Autodesk Inventor part; units mm, degrees
ref_plane "YZ Plane" through (0, 0, 0) normal (1, 0, 0) x (0, 1, 0)
ref_plane "XZ Plane" through (0, 0, 0) normal (0, 1, 0) x (-1, 0, 0)
ref_plane "XY Plane" through (0, 0, 0) normal (0, 0, 1) x (1, 0, 0)
sketch "スケッチ1" plane through (0, 0, 0) normal (0, 0, 1) x (1, 0, 0)
  line L0 (-17.75, 4) -> (17.75, 4)
  line L1 (17.75, 4) -> (17.75, -4)
  line L2 (17.75, -4) -> (-17.75, -4)
  line L3 (-17.75, -4) -> (-17.75, 4)
  line L4 (-17.75, 4) -> (17.75, -4) construction
  line L5 (17.75, 4) -> (-17.75, -4) construction
  point P0 (0, 0)
  dimension "d0" = 35.5
  dimension "d1" = 8
extrude "押し出し1" add sketch "スケッチ1" along normal mid plane 0.55
sketch "スケッチ2" plane through (0, 0, 0.275) normal (0, 0, 1) x (1, 0, 0)
  line L0 (9.6635, 0) -> (12.3865, 0) construction
  line L1 (9.6635, 1.3635) -> (12.3865, 1.3635)
  line L2 (12.3865, -1.3635) -> (9.6635, -1.3635)
  arc A0 (9.6635, 1.3635) -> (9.6635, -1.3635) centre (9.6635, 0) ccw
  arc A1 (12.3865, -1.3635) -> (12.3865, 1.3635) centre (12.3865, 0) ccw
  line L3 (17.75, -4) -> (17.75, 4)
  line L4 (17.75, 4) -> (-17.75, 4)
  point P0 (0, 0)
  point P1 (11.025, 0)
  point P2 (13.75, 0)
  point P3 (8.3, 0)
  dimension "d4" = 2.727
  dimension "d5" = 5.45
  dimension "d6" = 4
  dimension "d7" = 4
extrude "押し出し2" cut sketch "スケッチ2" against normal blind 0.55
sketch "スケッチ3" plane through (0, 0, 0.275) normal (0, 0, 1) x (1, 0, 0)
  line L0 (-17.75, 4) -> (17.75, 4)
  line L1 (17.75, 4) -> (17.75, -4)
  line L2 (-17.75, 4) -> (-17.75, -4)
  line L3 (-2.25, 3) -> (17.75, 3)
  line L4 (-3.75, 4) -> (-2.25, 3)
  line L5 (0, 0) -> (-1.8887, 0)
  line L6 (-2.25, -3) -> (17.75, -3)
  line L7 (-3.75, -4) -> (-2.25, -3)
  arc A0 (9.6635, 1.3635) -> (9.6635, -1.3635) centre (9.6635, 0) ccw
  line L8 (9.6635, 1.3635) -> (12.3865, 1.3635)
  arc A1 (12.3865, -1.3635) -> (12.3865, 1.3635) centre (12.3865, 0) ccw
  line L9 (12.3865, -1.3635) -> (9.6635, -1.3635)
  line L10 (-17.75, -4) -> (17.75, -4)
  line L11 (17.75, -4) -> (17.75, 4)
  line L12 (17.75, 4) -> (-17.75, 4)
  line L13 (-17.75, 4) -> (-17.75, -4)
  dimension "d10" = 1
  dimension "d11" = 14
  dimension "d12" = 20
extrude "押し出し3" cut sketch "スケッチ3" against normal blind 0.55 contours L0 L1 L3 L4 | L7 L6 L1 L10
sketch "スケッチ4" plane through (-17.75, -4, -0.275) normal (0, -1, 0) x (1, 0, 0)
  line L0 (0, 0.55) -> (14, 0.55)
  line L1 (0, 0.55) -> (0, 0)
  line L2 (0, 0) -> (1.6, 0.55)
  point P0 (17.75, 0.275)
  dimension "d15" = 1.6
extrude "押し出し4" cut sketch "スケッチ4" against normal through all
properties part number "pen_type_cutter"
Design review of the part built by this model. Coordinates are the model's own, in mm. A direction names the side the tool comes from. Round coordinates to 2 decimals unless told otherwise and drop trailing zeros. Write each loop counter-clockwise with the first axis right and the second up, starting at its lowest first coordinate (ties: lowest second). Pieces come first, ordered by that corner, then holes.
Item 1: We need section A-A on y = 0. Write out the cut boundary in (x, z) (3 decimals).
Item 2: The part is to be moulded in two halves that separate along X. For faces 1 (the flat face through (-16.961, -0.056, -0.004)), 2 (the cylindrical face through (13.75, -0.03, 0)), 3 (the flat face through (-3, 3.5, 0)), say which applies: +X half, -X half, draft (parallel to the pull), parting line (faces both ways), or undercut.
Item 3: For faces 4 (the flat face through (1, 0, 0.275)), 5 (the cylindrical face through (8.3, 0, 0)), list the 3-axis set-ups (+Z, -Z, +X, -X, +Y, -Y) from which the entire face can be reached by the end or side of a thin tool; tool diameter is ignored.
Item 4: For probe 1 along Y at (x, z) = (16.5, -0.2), list the stretches that pass through material, from the lowest coordinate up.
Item 5: We need section C-C on x = 14.5. Write out the cut boundary in (y, z) (3 decimals).
Item 6: We need section B-B on z = 0. Write out the cut boundary in (x, y).
Item 7: We need section D-D on y = -3.5. Write out the cut boundary in (x, z) (3 decimals).
Returned:
1. outline: (-17.75, -0.275) - (8.3, -0.275) - (8.3, 0.275) - (-16.15, 0.275) - close; (13.75, -0.275) - (17.75, -0.275) - (17.75, 0.275) - (13.75, 0.275) - close
2. face 1: -X half
2. face 2: undercut
2. face 3: +X half
3. face 4: +Z, +X, -X, +Y, -Y
3. face 5: +Z, -Z
4. probe 1: y = -3 to 3
5. outline: (-3, -0.275) - (3, -0.275) - (3, 0.275) - (-3, 0.275) - close
6. outline: (-16.95, -4) - (-3.75, -4) - (-2.25, -3) - (17.75, -3) - (17.75, 3) - (-2.25, 3) - (-3.75, 4) - (-16.95, 4) - close; hole (9.66, -1.36) - (12.39, -1.36) arc R1.36 ccw to (12.39, 1.36) - (9.66, 1.36) arc R1.36 ccw to start
7. outline: (-17.75, -0.275) - (-3, -0.275) - (-3, 0.275) - (-16.15, 0.275) - close
